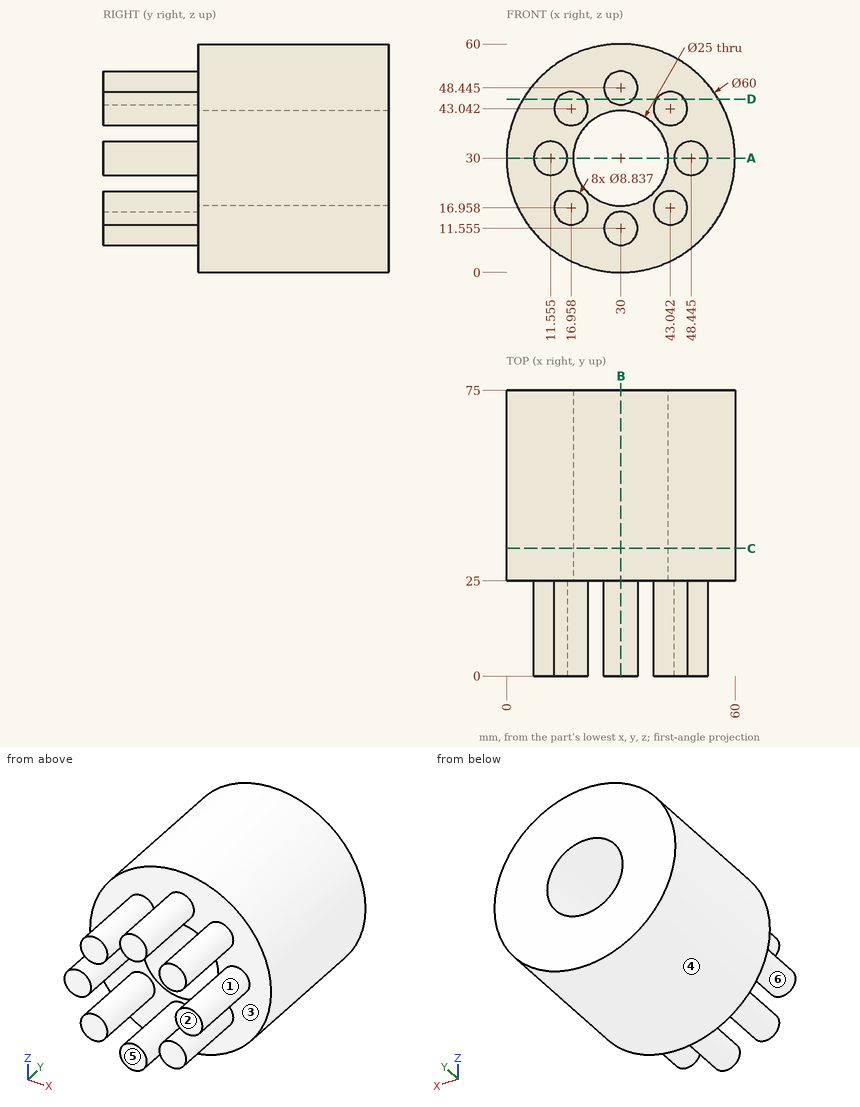
Study the drawing (mm; zero at the part's minimum x, y, z) and answer. A direction names the side the tool comes from. Give positions to 0.01 mm unless a question says otherwise; leave off trailing zeros. Order: outer loops, then holes, each group sorted by start corner. A loop starts at its lowest first (then second) coordinate and runs counter-clockwise, first axis right, second up. Notation, with made-up numbers: (4.25, 27) - (14.25, 27) arc R18 cw to (14.25, 42) - close; hole circle Ø6 at (-27.5, 68). An arc over 180 degrees is marked (long way). Answer in a Markdown table with one row per item. Add a question column.
Q1. Given P1, Ø4, axis at x = 13.5, y = 60.5, coming from the +Z side; P2, Ø12, axis at x = 49.5, y = 65, coming from the +Z side; P3, Ø2, axis at x = 53.5, y = 15.5, coming from the +Z side (1 decimal), each flat-ended and moving along its own axis, determine where each tip first touches the part or whether it passes through.
Q2. The part is cut by section B-B (x = 30). Determine the outline of the cut face in (y, z), then the cut area to 3 significant figures.
Q3. Which of the six approach directions +Z, -Z, +X, -X, +Y, -Y give full straight-line access (tool end or side, diameter ignored) to the marked faces 1 and 2?
Q4. The part is cut by section D-D (z = 45.5). Determine the outline of the cut face in (x, y) (1 decimal), then the cut area to 3 significant figures.
Q5. The part is cut by section C-C (y = 33.5). Determine the outline of the cut face in (x, z).
Q6. For a pull along X with two mould halves and no side action, classify the marked faces 3, 4, 5 and 6 as released by +X, released by -X, zero draft, split by the parting line, or undercut.
Q7. Find the intervals of material crossed by line 1 along Z through (x, y) = (30, 63); line 2 along Z through (x, y) = (44.5, 20) (1 decimal); line 3 along Y through (x, z) = (27, 53), in increasing order. Write a range as [from, to].
Q8. The part is cut by section A-A (z = 30). Determine the outline of the cut face in (x, y).
Determined:
| question | item | result |
|---|---|---|
| 1 | P1 | stops at z = 56.26 |
| 1 | P2 | stops at z = 56.79 |
| 1 | P3 | stops at z = 31.8 |
| 2 | outline | (0, 7.14) - (25, 7.14) - (25, 0) - (75, 0) - (75, 17.5) - (25, 17.5) - (25, 15.97) - (0, 15.97) - close; (0, 44.03) - (25, 44.03) - (25, 42.5) - (75, 42.5) - (75, 60) - (25, 60) - (25, 52.86) - (0, 52.86) - close |
| 2 | area | 2,190 mm² |
| 3 | face 1 | -Y |
| 3 | face 2 | +Z, -Z, +X, -X, -Y |
| 4 | outline | (4.3, 25) - (13.3, 25) - (13.3, 0) - (20.6, 0) - (20.6, 25) - (26.7, 25) - (26.7, 0) - (33.3, 0) - (33.3, 25) - (39.4, 25) - (39.4, 0) - (46.7, 0) - (46.7, 25) - (55.7, 25) - (55.7, 75) - (4.3, 75) - close |
| 4 | area | 3,100 mm² |
| 5 | outline | circle Ø60 at (30, 30); hole circle Ø25 at (30, 30) |
| 6 | face 3 | undercut |
| 6 | face 4 | split by the parting line |
| 6 | face 5 | zero draft |
| 6 | face 6 | undercut |
| 7 | line 1 | z = [0, 17.5], [42.5, 60] |
| 7 | line 2 | z = [12.8, 21.1], [28, 32], [38.9, 47.2] |
| 7 | line 3 | y = [25, 75] |
| 8 | outline | (0, 25) - (7.14, 25) - (7.14, 0) - (15.97, 0) - (15.97, 25) - (17.5, 25) - (17.5, 75) - (0, 75) - close; (42.5, 25) - (44.03, 25) - (44.03, 0) - (52.86, 0) - (52.86, 25) - (60, 25) - (60, 75) - (42.5, 75) - close |
